Answer from the drawing. Dimensions are ordinates in mm from the lowest x, y and z of the part. A direction names the side the tool comes from. Coordinates: 2 decimals unless noted, no trailing zeros. Write each loop counter-clockwise with the first axis right and the second up, starting at its lowest first coordinate (ties: lowest second). Pieces come first, ordered by that corner, then holes. Notation, with made-up numbers: (62.5, 34) - (110.5, 34) arc R35 ccw to (110.5, 66) - close; hole circle Ø11 at (55, 85). An arc over 180 degrees is marked (long way). Answer as a JSON object with one key per item and string values. Group by question number.
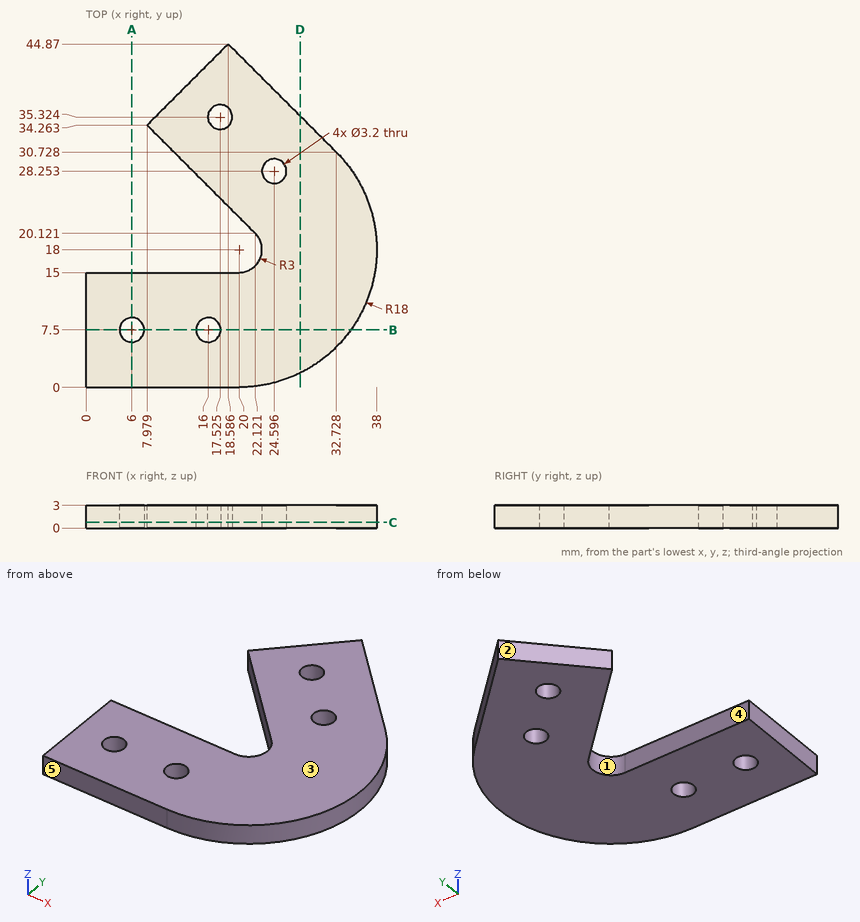
Q1. Consider L1, parallel to Y at x = 6, z = 1.1; L2, parallel to Y at x = 20, z = 2.8 (1 decimal); L3, parallel to X at y = 34.5, z = 0.5 (1 decimal). Determine where each line is inside the solid, lowest interval first. Write a range as from..to.
Q2. Section B-B on y = 7.5 is taken. Determine the outline of the cut face in (x, z).
Q3. Section A-A on x = 6 is taken. Determine the outline of the cut face in (y, z).
Q4. For a pull along Y with two mould halves and no side action, classify the marked faces 1, 2 and 3 as +Y half, -Y half, draft (parallel to the pull), parting line (faces both ways), or undercut.
Q5. A tool of negligible diameter and unlimited length cuts with its end or side. For the marked faces 4 and 5, from which of +Z, -Z, +X, -X, +Y, -Y can it reach the whole face along a straight path? Write none if from no direction.
Q6. Section C-C on z = 0.75 is taken. Determine the outline of the cut face in (x, y) (1 decimal), plus the area to 3 significant figures.
Q7. Section D-D on x = 28 is taken. Determine the outline of the cut face in (y, z) (1 decimal).
Q8. Flat-ended cylindrical pins translate along their axes: pin 1 Ø1.9 at (x, y) = (6, 7.5) entering from -Z; pin 2 Ø0.9 at (x, z) = (11.5, 2) entering from +Y (1 decimal). Find the tip coordinate at first contact, or state that the pin passes through.
Numbers:
{
 "1": {"L1": "y = 0..5.9, 9.1..15", "L2": "y = 0..15, 22.2..43.5", "L3": "x = 8.2..16.2, 18.9..29"},
 "2": {"outline": "(0, 0) - (4.4, 0) - (4.4, 3) - (0, 3) - close; (7.6, 0) - (14.4, 0) - (14.4, 3) - (7.6, 3) - close; (17.6, 0) - (34.62, 0) - (34.62, 3) - (17.6, 3) - close"},
 "3": {"outline": "(0, 0) - (5.9, 0) - (5.9, 3) - (0, 3) - close; (9.1, 0) - (15, 0) - (15, 3) - (9.1, 3) - close"},
 "4": {"face 1": "undercut", "face 2": "+Y half", "face 3": "draft"},
 "5": {"face 4": "+Z, -Z, -X", "face 5": "+Z, -Z, +X, -X, -Y"},
 "6": {"outline": "(0, 0) - (20, 0) arc R18 ccw to (32.7, 30.7) - (18.6, 44.9) - (8, 34.3) - (22.1, 20.1) arc R3 cw to (20, 15) - (0, 15) - close; hole circle Ø3.2 at (6, 7.5); hole circle Ø3.2 at (16, 7.5); hole circle Ø3.2 at (17.5, 35.3); hole circle Ø3.2 at (24.6, 28.3)", "area": "939 mm²"},
 "7": {"outline": "(1.9, 0) - (35.5, 0) - (35.5, 3) - (1.9, 3) - close"},
 "8": {"pin 1": "passes through", "pin 2": "stops at y = 38.2"}
}
